Geometry: final body of the model. Coordinates: model frame, mm. Face numbers are marked on the shaded views. A direction names the side the tool comes from. Round coordinates to 2 decimals unless told otherwise and drop trailing zeros. Loops run counter-clockwise (first coordinate to the right, second up) from the corner with the lowest first, then second, coordinate; pieces in that order, holes last. Notation, with made-up numbers: (-33, 12) - (1, 12) arc R30 cw to (1, 51) - close; hole circle Ø1 at (48, 28.5). An arc over 180 degrees is marked (long way). Answer in a Markdown table with one row per item. Add a question column.
from build123d import *

# Parameters (mm, degrees)
SKETCH_1_R          = 16
EXTRUDE_1_DEPTH     = 8
SKETCH_2_R          = 7
EXTRUDE_2_DEPTH     = 2
SKETCH_3_R          = 2
CUT_EXTRUDE_1_DEPTH = 20
SKETCH_4_R          = 3
CUT_EXTRUDE_2_DEPTH = 20


with BuildPart() as part:
    # 草图1 → 凸台-拉伸1 (new body)
    with BuildSketch(Plane.XY):
        Circle(SKETCH_1_R)
    extrude(amount=EXTRUDE_1_DEPTH)

    # 草图2 → 凸台-拉伸2 (add)
    with BuildSketch(Plane.XY.offset(8)):
        Circle(SKETCH_2_R)
    extrude(amount=EXTRUDE_2_DEPTH)

    # 草图3 → 切除-拉伸1 (cut)
    with BuildSketch(Plane.XY.offset(8)):
        with Locations((-8, 8)):
            Circle(SKETCH_3_R)
        with Locations((8, 8)):
            Circle(SKETCH_3_R)
        with Locations((8, -8)):
            Circle(SKETCH_3_R)
        with Locations((-8, -8)):
            Circle(SKETCH_3_R)
    extrude(amount=-CUT_EXTRUDE_1_DEPTH, mode=Mode.SUBTRACT)

    # 草图4 → 切除-拉伸2 (cut)
    with BuildSketch(Plane.XY.offset(10)):
        Circle(SKETCH_4_R)
    extrude(amount=-CUT_EXTRUDE_2_DEPTH, mode=Mode.SUBTRACT)


solid = part.part
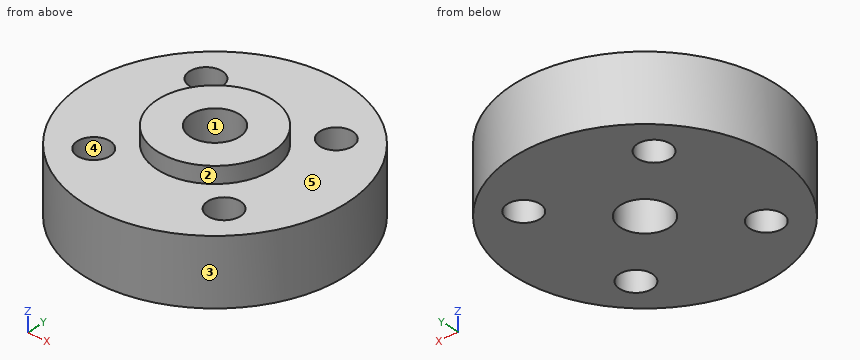
1) Section B-B, the plane z = 5.25. Return the cut outline in (x, y).
2) Pull-direction query (Y, two-part tool) for the marked faces 3, 4 and 5; classes: pulls with the +Y half, pulls with the -Y half, needs draft (parallel to the pull), parting line crosses it, or undercut.
3) Material intervals for line 1 along Y through (x, z) = (-8, 2); line 2 along X through (y, z) = (6.5, 2.25); line 3 along Z through (x, y) = (-9, 4.5), sorted ascending. Write a range as from..to.
4) Section D-D, the plane x = -8.5. Return the cut outline in (y, z), and give its area (3 significant figures).
5) Reachability of the marked faces 1 and 2 from +Z, -Z, +X, -X, +Y, -Y: full face, straight path, thin tool, end or side. Return the list, or none.
6) Section A-A, the plane x = 0. Return the cut outline in (y, z).
7) Contact query for flat-ended pins moving along their axis: pin 1 Ø1 at (y, z) = (-10.5, 3.5) entering from +X; pin 2 Ø6.5 at (x, y) = (8, -8) entering from +Z; pin 3 Ø16 at (x, y) = (-6.5, 4) entering from +Z; pin 4 Ø5 at (x, z) = (3.5, 3) entering from +Y. Output: stop coordinate, or through.
8) Section C-C, the plane y = -9.5. Return the cut outline in (x, z), and give its area (3 significant figures).
Evaluation:
| question | item | result |
|---|---|---|
| 1 | outline | circle Ø32 at (0, 0); hole circle Ø4 at (-8, -8); hole circle Ø4 at (-8, 8); hole circle Ø6 at (0, 0); hole circle Ø4 at (8, -8); hole circle Ø4 at (8, 8) |
| 2 | face 3 | parting line crosses it |
| 2 | face 4 | undercut |
| 2 | face 5 | needs draft |
| 3 | line 1 | y = -13.86..-10, -6..6, 10..13.86 |
| 3 | line 2 | x = -14.62..-9.32, -6.68..6.68, 9.32..14.62 |
| 3 | line 3 | z = 0..8 |
| 4 | outline | (-13.56, 0) - (-9.94, 0) - (-9.94, 8) - (-13.56, 8) - close; (-6.06, 0) - (6.06, 0) - (6.06, 8) - (-6.06, 8) - close; (9.94, 0) - (13.56, 0) - (13.56, 8) - (9.94, 8) - close |
| 4 | area | 155 mm² |
| 5 | face 1 | +Z, -Z |
| 5 | face 2 | +Z |
| 6 | outline | (-16, 0) - (-3, 0) - (-3, 10) - (-7, 10) - (-7, 8) - (-16, 8) - close; (3, 0) - (16, 0) - (16, 8) - (7, 8) - (7, 10) - (3, 10) - close |
| 7 | pin 1 | stops at x = 12.49 |
| 7 | pin 2 | stops at z = 8 |
| 7 | pin 3 | stops at z = 10 |
| 7 | pin 4 | stops at y = 15.97 |
| 8 | outline | (-12.87, 0) - (-9.32, 0) - (-9.32, 8) - (-12.87, 8) - close; (-6.68, 0) - (6.68, 0) - (6.68, 8) - (-6.68, 8) - close; (9.32, 0) - (12.87, 0) - (12.87, 8) - (9.32, 8) - close |
| 8 | area | 164 mm² |
